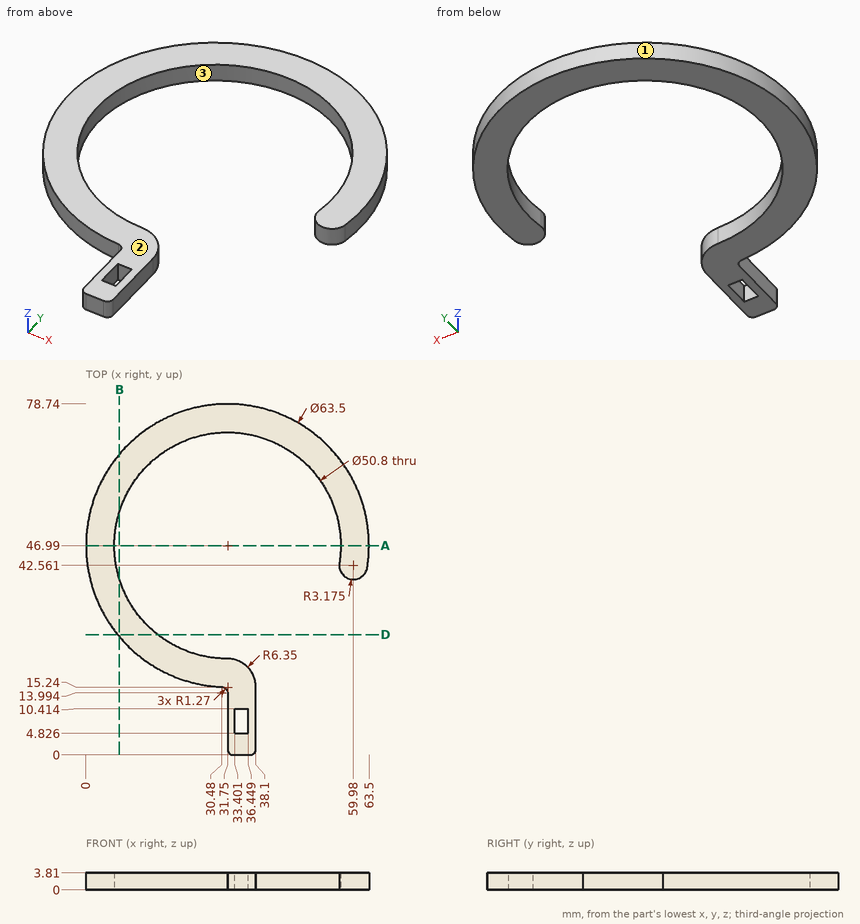
The figure shows three views and two pictorial views of one solid part (mm, origin at its lowest corner). Answer the questions. Give positions to 0.01 mm unless a question says otherwise; leave off trailing zeros. Loops run counter-clockwise (first coordinate to the right, second up) from the corner with the lowest first, then second, coordinate; pieces in that order, holes last. Notation, with made-up numbers: (9, 35) -> (35, 35) arc R10 cw to (35, 43) -> close; hole circle Ø6 at (24, 35.25). An arc over 180 degrees is marked (long way). Put each result on its own line as item: value. Start each with the question number.
Item 1: The part is cut by section B-B (x = 7.5). Give the vertices of the cut face in (y, z).
Item 2: The mould has two halves that part along Y. Classify the marked faces 1, 2 and 3: released by +Y, released by -Y, zero draft, split by the parting line, or undercut.
Item 3: Find the intervals of material crossed by L1, parallel to X at y = 46.99, z = 2.4; L2, parallel to Y at x = 35, z = 0.25 (1 decimal); L3, parallel to X at y = 54.5, z = 3.3 (1 decimal), in increasing order. Write a range as [from, to].
Item 4: The part is cut by section A-A (y = 46.99). Give the vertices of the cut face in (x, z).
Item 5: The part is cut by section D-D (y = 27). Give the vertices of the cut face in (x, z), then the cut area to 3 significant figures.
Item 6: Each of these flat-tipped pins is pushed along its axis until it touches: P1, Ø2, axis at x = 48, z = 3.5, coming from the -Y side (1 decimal); P2, Ø1.1, axis at y = 10.5, z = 2, coming from the +X side; P3, Ø1.9, axis at y = 6, z = 1.5, coming from the -X side. Where does it stop, or does it pass through?
Answers below:
1. outline: (26.5, 0) -> (39.43, 0) -> (39.43, 3.81) -> (26.5, 3.81) -> close; (54.55, 0) -> (67.48, 0) -> (67.48, 3.81) -> (54.55, 3.81) -> close
2. face 1: split by the parting line
2. face 2: zero draft
2. face 3: undercut
3. L1: [0, 6.35], [57.15, 63.5]
3. L2: [0, 4.8], [10.4, 20.7], [72.2, 78.6]
3. L3: [0.9, 7.5], [56, 62.6]
4. outline: (0, 0) -> (6.35, 0) -> (6.35, 3.81) -> (0, 3.81) -> close; (57.15, 0) -> (63.5, 0) -> (63.5, 3.81) -> (57.15, 3.81) -> close
5. outline: (7.08, 0) -> (16.08, 0) -> (16.08, 3.81) -> (7.08, 3.81) -> close
5. area: 34.3 mm2
6. P1: y = 65.6
6. P2: x = 38.1
6. P3: x = 31.75
